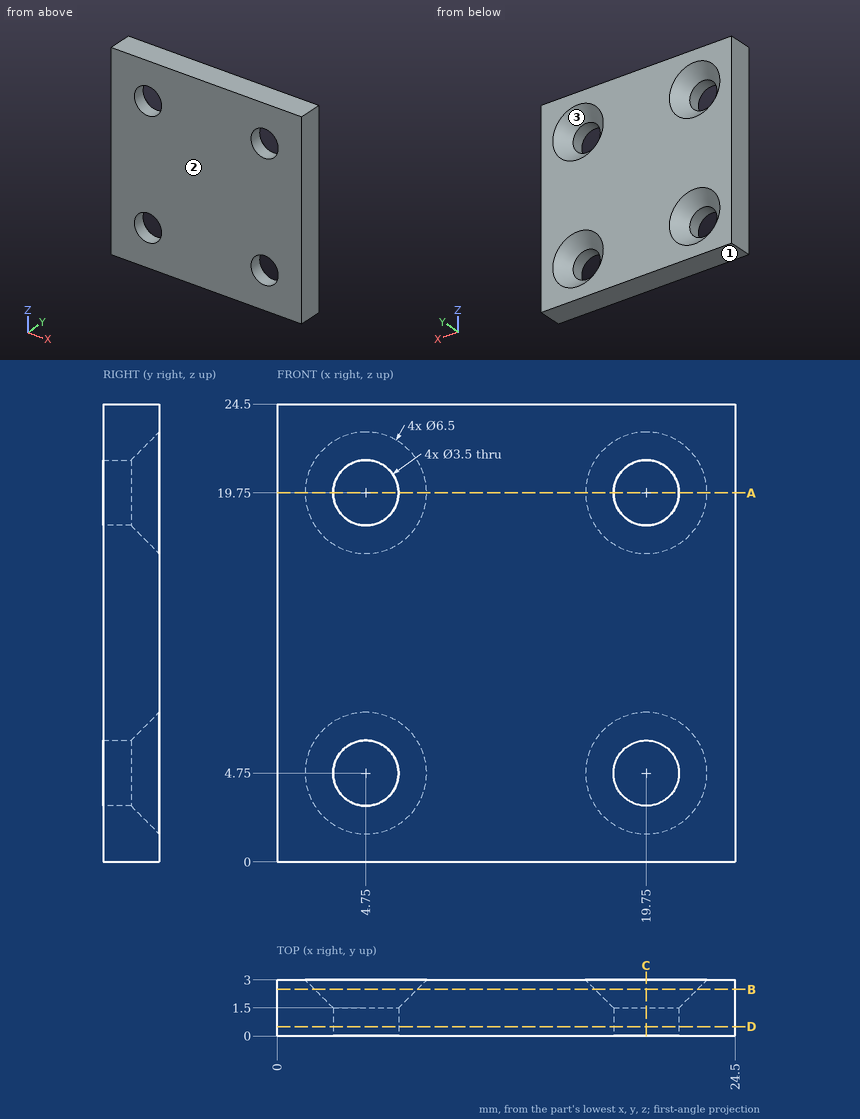
Could you check a few things on this drawing? It's one solid part, dimensions in mm from its lowest x, y, z. Coordinates: 2 decimals unless noted, no trailing zeros. Write each loop counter-clockwise with the first axis right and the second up, starting at its lowest first coordinate (ties: lowest second). Pieces come first, ordered by that corner, then holes.
1) If we section it at B-B (y = 2.5): List the corners of the cut face in (x, z) for me.
Filled in:
outline: (0, 0) - (24.5, 0) - (24.5, 24.5) - (0, 24.5) - close; hole circle Ø5.5 at (4.75, 4.75); hole circle Ø5.5 at (4.75, 19.75); hole circle Ø5.5 at (19.75, 4.75); hole circle Ø5.5 at (19.75, 19.75)
2) Thinking about a two-plate mould opening in Z: for the marked faces 1, 2 and 3, which applies, +Z half, -Z half, draft (parallel to the pull), parting line (faces both ways), or undercut?
Filled in:
face 1: -Z half
face 2: draft
face 3: undercut
3) If I drill on line 1 (X direction, y = 0.3, z = 19.75); line 2 (Z direction, x = 6, y = 0.55); line 3 (Z direction, x = 3.25, y = 0.95), over which ranges is the centre line in solid material (lowest first)?
Filled in:
line 1: x = 0 to 3, 6.5 to 18, 21.5 to 24.5
line 2: z = 0 to 3.53, 5.97 to 18.53, 20.97 to 24.5
line 3: z = 0 to 3.85, 5.65 to 18.85, 20.65 to 24.5
4) If we section it at A-A (z = 19.75): List the corners of the cut face in (x, y) for me.
Filled in:
outline: (0, 0) - (3, 0) - (3, 1.5) - (1.5, 3) - (0, 3) - close; (6.5, 0) - (18, 0) - (18, 1.5) - (16.5, 3) - (8, 3) - (6.5, 1.5) - close; (21.5, 0) - (24.5, 0) - (24.5, 3) - (23, 3) - (21.5, 1.5) - close
5) If we section it at C-C (x = 19.75): List the corners of the cut face in (y, z) for me, plus the area to 3 significant figures.
Filled in:
outline: (0, 0) - (3, 0) - (3, 1.5) - (1.5, 3) - (0, 3) - close; (0, 6.5) - (1.5, 6.5) - (3, 8) - (3, 16.5) - (1.5, 18) - (0, 18) - close; (0, 21.5) - (1.5, 21.5) - (3, 23) - (3, 24.5) - (0, 24.5) - close
area: 48.0 mm2
6) I'm going to push a flat-ended pin straight in: pin 1 (4 mm diameter, centred on x = 4.75, z = 4.75, fed in from +Y). Where does the tip first touch, or does it pass through?
Filled in:
pin 1: stops at y = 1.75
7) If we section it at D-D (y = 0.5): List the corners of the cut face in (x, z) for me.
Filled in:
outline: (0, 0) - (24.5, 0) - (24.5, 24.5) - (0, 24.5) - close; hole circle Ø3.5 at (4.75, 4.75); hole circle Ø3.5 at (4.75, 19.75); hole circle Ø3.5 at (19.75, 4.75); hole circle Ø3.5 at (19.75, 19.75)
